Autodesk Inventor part; units mm, degrees
ref_plane "YZ Plane" through (0, 0, 0) normal (1, 0, 0) x (0, 1, 0)
ref_plane "XZ Plane" through (0, 0, 0) normal (0, 1, 0) x (-1, 0, 0)
ref_plane "XY Plane" through (0, 0, 0) normal (0, 0, 1) x (1, 0, 0)
sketch "Sketch1" plane through (0, 0, 0) normal (0, 0, 1) x (1, 0, 0)
  circle A0 centre (0, 0) radius 4
  dimension "Diameter" = 8
extrude "Extrusion1" add sketch "Sketch1" along normal blind 15
sketch "Sketch2" plane through (0, 0, 15) normal (0, 0, 1) x (1, 0, 0)
  circle A0 centre (0, 0) radius 4
  circle A1 centre (0, 0) radius 6.5
  dimension "Head_Diameter" = 13
extrude "Extrusion2" add sketch "Sketch2" along normal blind 8 contours A0 | A1
sketch "Sketch3" plane through (0, 0, 23) normal (0, 0, 1) x (1, 0, 0)
  circle A0 centre (0, 0) radius 6.5
  circle A1 centre (0, 0) radius 3.4641 construction
  line L0 (0, 3.4641) -> (3, 1.7321)
  line L1 (3, -1.7321) -> (3, 1.7321)
  line L2 (0, 3.4641) -> (-3, 1.7321)
  line L3 (-3, -1.7321) -> (-3, 1.7321)
  line L4 (-3, -1.7321) -> (0, -3.4641)
  line L5 (3, -1.7321) -> (0, -3.4641)
  dimension "Hex_Width" = 6
extrude "Extrusion3" cut sketch "Sketch3" against normal blind 4 contours L0 L1 L5 L4 L3 L2
thread "Thread1"
chamfer "Chamfer1" distance 0.8 angle 45 2 edges at (-6.5, 0, 23) (-4, 0, 0)
equation "\"d9\" = ThreadLength"
equation "\"d12\" = Chamfer"
equation "\"ThreadLength\" = 15"
properties part number "SCREW, SOCKET HD, P, 12.9, M8X1.25X15MM"
Geometry check sheet. Reference: the model listing, model coordinates, mm. A direction names the side the tool comes from. Give positions to 0.01 mm unless a question says otherwise; leave off trailing zeros. Loops run counter-clockwise (first coordinate to the right, second up) from the corner with the lowest first, then second, coordinate; pieces in that order, holes last. Notation, with made-up numbers: M 27,1 L 32,1 A34 cw 32,34 Z; hole C 56,38.5 d9. An arc over 180 degrees is marked long. Answer as CSV lines item,"result".
Item 1: Cross-section at B-B on z = 10.25. Record the cut outline in (x, y), and give its area (3 significant figures).
Values:
outline,"C 0,0 d8"
area,"50.3 mm²"
Item 2: Depth check by flat-ended pin: P1, Ø5, axis at y = -1.5, z = 7.5, coming from the -X side; P2, Ø1.5, axis at y = 4, z = 10.5, coming from the +X side; P3, Ø6, axis at y = 3, z = 19, coming from the +X side; P4, Ø5, axis at y = 2.5, z = 13, coming from the -X side. Enter the tip coordinate at first touch or a pass-through.
Values:
P1,"stops at x = -4"
P2,"stops at x = 2.33"
P3,"stops at x = 6.5"
P4,"stops at x = -6.42"
Item 3: Access from +Z, -Z, +X, -X, +Y, -Y to the whole of each face (thin tool, end or side, straight path). Record for faces 1 (the flat face through (-3, 0, 21)), 2 (the flat face through (3, 3, 15)), 3 (the flat face through (0, 0, 0)).
Values:
face 1,"+Z"
face 2,"-Z"
face 3,"-Z, +X, -X, +Y, -Y"
Item 4: Release check for a two-part mould opening along Y. For faces 4 (the cylindrical face through (-5.158, 3.955, 18.55)), 5 (the flat face through (0, 0, 19)), 6 (the flat face through (2.5, -2.5, 23)), 7 (the flat face through (-1.5, 2.6, 21)) record: pulls with the +Y half, pulls with the -Y half, needs draft (parallel to the pull), parting line crosses it, or undercut.
Values:
face 4,"parting line crosses it"
face 5,"undercut"
face 6,"needs draft"
face 7,"undercut"
Item 5: Cross-section at A-A on y = 0. Record the cut outline in (x, z).
Values:
outline,"M -6.5,15 L -4,15 L -4,0.8 L -3.2,0 L 3.2,0 L 4,0.8 L 4,15 L 6.5,15 L 6.5,22.2 L 5.7,23 L 3,23 L 3,19 L -3,19 L -3,23 L -5.7,23 L -6.5,22.2 Z"
Item 6: Material ranges on line 1 (Z direction, x = 5.5, y = -0.5); line 2 (X direction, y = 1, z = 20.5); line 3 (X direction, y = -0.25, z = 17.75), recorded low to high.
Values:
line 1,"z = 15 to 23"
line 2,"x = -6.42 to -3, 3 to 6.42"
line 3,"x = -6.5 to 6.5"
